Part model, mm, in its own coordinate system. Round coordinates to 2 decimals unless told otherwise and drop trailing zeros. Write each loop counter-clockwise with the first axis right and the second up, starting at its lowest first coordinate (ties: lowest second). Pieces come first, ordered by that corner, then holes.
1) Saw through at B-B on y = -1.6. Write the cut outline in (x, z).
2) Saw through at A-A on x = 0. Write the cut outline in (y, z).
3) Drill centre lines: L1, parallel to Z at x = 0, y = -1.45; L2, parallel to Z at x = -0.25, y = -1.05; L3, parallel to X at y = -1.35, z = 44. Where is each one in solid material? Low to high.
4) Pull direction X, two halves, no side cores. Call faces 1 (the cylindrical face through (-0.33, -0.99, -26.28)), 2 (the flat face through (5, -1, 8)), 3 (the cylindrical face through (-0.52, -0.99, -6.08)), 4 (the flat face through (0, 0, 9)): +X half, -X half, draft (parallel to the pull), parting line (faces both ways), or undercut.
5) Saw through at D-D on x = 4. Write the cut outline in (y, z).
6) Saw through at C-C on z = 45.5. Write the cut outline in (x, y), and give its area (3 significant figures).
7) Flat gauge pins, fed straight in: pin 1 (6 mm diameter, centred on x = 0, z = 46.24, fed in from -Y); pin 2 (1 mm diameter, centred on x = 3, y = -1.5, fed in from +Z); pin 3 (4.5 mm diameter, centred on x = 0, z = -28.76, fed in from -Y). Where does each tip first touch, or does it go through?
```python
from build123d import *

# Parameters (mm, degrees)
F0_R     = 2.5
F0_R_2   = 2.378566
F1_DEPTH = 2


with BuildPart() as f1:
    # F0 (on Front) → F1 (new body)
    with BuildSketch(Plane.XZ):
        with BuildLine():
            Line((5, -28.759506), (5, 46.240494))
            ThreePointArc((5, 46.240494), (0, 51.240494), (-5, 46.240494))
            Line((-5, 46.240494), (-5, -28.759506))
            ThreePointArc((-5, -28.759506), (0, -33.759506), (5, -28.759506))
        make_face()
        with Locations((0, -28.759506)):
            Circle(F0_R, mode=Mode.SUBTRACT)
        with Locations((0, -3.759506)):
            Circle(F0_R_2, mode=Mode.SUBTRACT)
        with Locations((0, 46.240494)):
            Circle(F0_R, mode=Mode.SUBTRACT)
    extrude(amount=F1_DEPTH)


solid = f1.part
```
Completed:
1. outline: (-5, -28.76) arc R5 ccw to (5, -28.76) - (5, 46.24) arc R5 ccw to (-5, 46.24) - close; hole circle Ø5 at (0, -28.76); hole circle Ø5 at (0, 46.24); hole circle Ø4.76 at (0, -3.76)
2. outline: (-2, -33.76) - (0, -33.76) - (0, -31.26) - (-2, -31.26) - close; (-2, -26.26) - (0, -26.26) - (0, -6.14) - (-2, -6.14) - close; (-2, -1.38) - (0, -1.38) - (0, 43.74) - (-2, 43.74) - close; (-2, 48.74) - (0, 48.74) - (0, 51.24) - (-2, 51.24) - close
3. L1: z = -33.76 to -31.26, -26.26 to -6.14, -1.38 to 43.74, 48.74 to 51.24
3. L2: z = -33.75 to -31.25, -26.27 to -6.12, -1.39 to 43.75, 48.73 to 51.23
3. L3: x = -5 to -1.11, 1.11 to 5
4. face 1: undercut
4. face 2: +X half
4. face 3: undercut
4. face 4: draft
5. outline: (-2, -31.76) - (0, -31.76) - (0, 49.24) - (-2, 49.24) - close
6. outline: (-5, -2) - (-2.39, -2) - (-2.39, 0) - (-5, 0) - close; (2.39, -2) - (5, -2) - (5, 0) - (2.39, 0) - close
6. area: 10.4 mm2
7. pin 1: stops at y = -2
7. pin 2: stops at z = 50.57
7. pin 3: passes through
